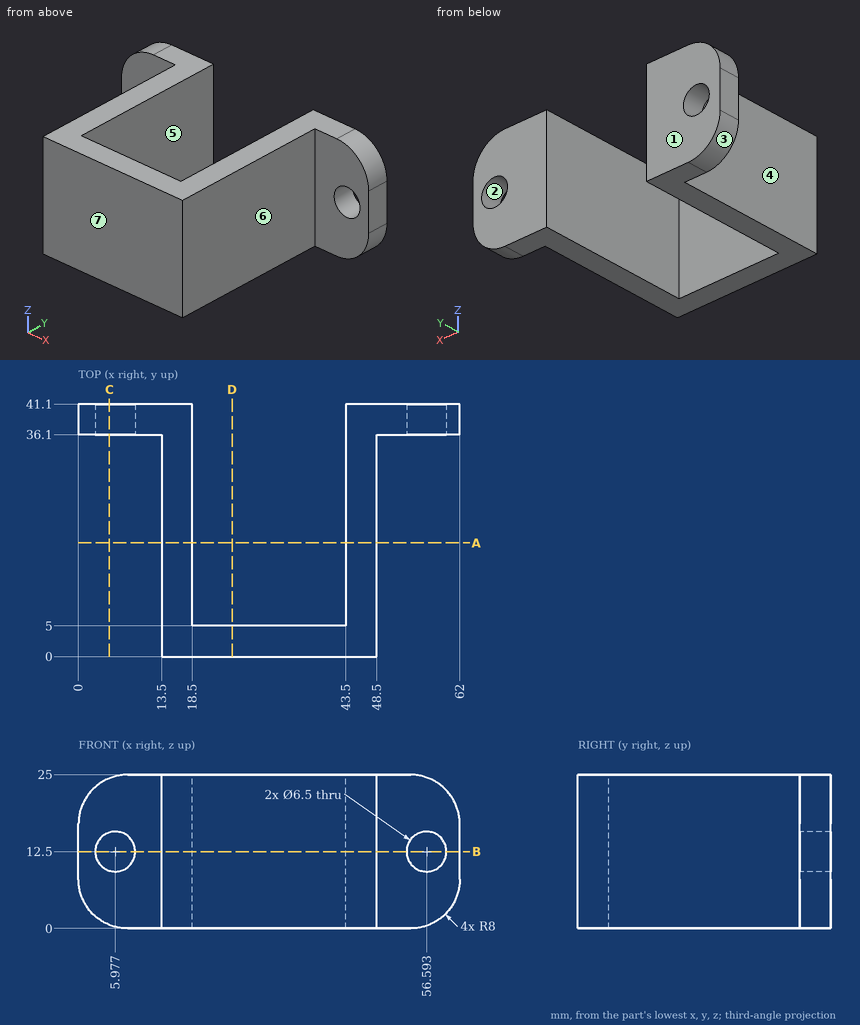
Check sheet for the drawn part. Datum: minimum x, y, z corner. Units: mm. A direction names the side the tool comes from. Round coordinates to 2 decimals unless told otherwise and drop trailing zeros. Order: outer loops, then holes, each group sorted by start corner. A loop starts at its lowest first (then second) coordinate and runs counter-clockwise, first axis right, second up.
1. Section check B-B on z = 12.5. Record the cut outline in (x, y), then the cut area to 3 significant figures.
Final values:
outline: (0, 36.1) - (2.73, 36.1) - (2.73, 41.1) - (0, 41.1) - close; (9.23, 36.1) - (13.5, 36.1) - (13.5, 0) - (48.5, 0) - (48.5, 36.1) - (53.34, 36.1) - (53.34, 41.1) - (43.5, 41.1) - (43.5, 5) - (18.5, 5) - (18.5, 41.1) - (9.23, 41.1) - close; (59.84, 36.1) - (62, 36.1) - (62, 41.1) - (59.84, 41.1) - close
area: 606 mm2
2. Section check A-A on y = 18.5. Record the cut outline in (x, z).
Final values:
outline: (13.5, 0) - (18.5, 0) - (18.5, 25) - (13.5, 25) - close; (43.5, 0) - (48.5, 0) - (48.5, 25) - (43.5, 25) - close
3. Section check D-D on x = 25. Record the cut outline in (y, z).
Final values:
outline: (0, 0) - (5, 0) - (5, 25) - (0, 25) - close
4. Release check for a two-part mould opening along X. For the marked faces 1, 2 and 3 record: +X half, -X half, draft (parallel to the pull), parting line (faces both ways), or undercut.
Final values:
face 1: draft
face 2: undercut
face 3: -X half
5. Access from +Z, -Z, +X, -X, +Y, -Y to the whole of each face (thin tool, end or side, straight path). Record for the marked faces 4, 5, 6 and 7.
Final values:
face 4: +Z, -Z, -X, -Y
face 5: +Z, -Z, +Y
face 6: +Z, -Z, +X, -Y
face 7: +Z, -Z, +X, -X, -Y
6. Go/stop test with flat-tipped pins: P1, Ø11, axis at x = 4, z = 18.5, coming from the -Y side; P2, Ø6, axis at y = 15.5, z = 5, coming from the -X side; P3, Ø5, axis at x = 38.5, z = 18.5, coming from the +Y side. Record where each tip stops, or that it passes through.
Final values:
P1: stops at y = 36.1
P2: stops at x = 13.5
P3: stops at y = 5
7. Section check C-C on x = 5. Record the cut outline in (y, z).
Final values:
outline: (36.1, 0.58) - (41.1, 0.58) - (41.1, 9.4) - (36.1, 9.4) - close; (36.1, 15.6) - (41.1, 15.6) - (41.1, 24.42) - (36.1, 24.42) - close
8. Thickness scan on L1, parallel to X at y = 24, z = 23.25; L2, parallel to Y at x = 27, z = 21.25; L3, parallel to Y at x = 55.5, z = 7.75. Record the ranges inside material, lowest first.
Final values:
L1: x = 13.5 to 18.5, 43.5 to 48.5
L2: y = 0 to 5
L3: y = 36.1 to 41.1
